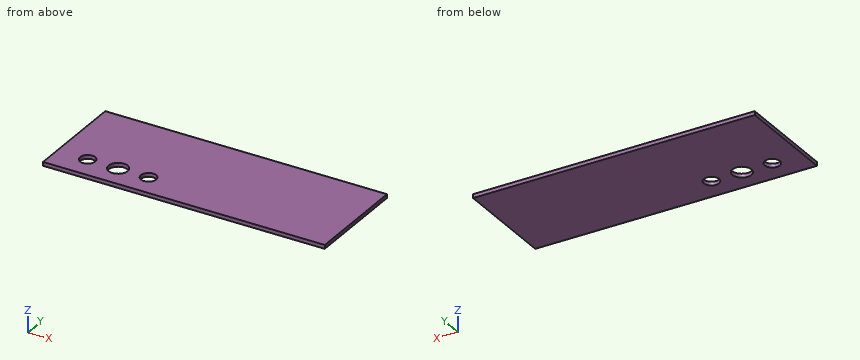
```python
from build123d import *

# Parameters (mm, degrees)
SKETCH1_W          = 234.95
SKETCH1_H          = 86.36
BASE_FLANGE1_DEPTH = 3.175
SKETCH11_R         = 7.9375
CUT_EXTRUDE3_DEPTH = 126.199715056
SKETCH13_R         = 6.35
CUT_EXTRUDE5_DEPTH = 126.199715056
SKETCH14_R         = 6.35
CUT_EXTRUDE6_DEPTH = 126.199715056


# Sheet-metal steps are written as plain solids
with BuildPart() as part:
    # Sketch1 → Base-Flange1 (new body)
    with BuildSketch(Plane.XY):
        Rectangle(SKETCH1_W, SKETCH1_H)
    extrude(amount=-BASE_FLANGE1_DEPTH)

    # Sketch11 → Cut-Extrude3 (cut, through all)
    with BuildSketch(Plane.XY):
        with Locations((-66.675, -23.495)):
            Circle(SKETCH11_R)
    extrude(amount=-CUT_EXTRUDE3_DEPTH, mode=Mode.SUBTRACT)

    # Sketch13 → Cut-Extrude5 (cut, through all)
    with BuildSketch(Plane.XY):
        with Locations((-41.275, -23.495)):
            Circle(SKETCH13_R)
    extrude(amount=-CUT_EXTRUDE5_DEPTH, mode=Mode.SUBTRACT)

    # Sketch14 → Cut-Extrude6 (cut, through all)
    with BuildSketch(Plane.XY):
        with Locations((-92.075, -23.495)):
            Circle(SKETCH14_R)
    extrude(amount=-CUT_EXTRUDE6_DEPTH, mode=Mode.SUBTRACT)


solid = part.part
```
Geometry: final body of the model. Coordinates: model frame, mm. Round coordinates to 2 decimals unless told otherwise and drop trailing zeros. Order: outer loops, then holes, each group sorted by start corner. A loop starts at its lowest first (then second) coordinate and runs counter-clockwise, first axis right, second up. Notation, with made-up numbers: (84, -27.5) -> (99, -27.5) arc R23 ccw to (99, 8.5) -> close; hole circle Ø9 at (78, -20.5). An arc over 180 degrees is marked (long way). Use one line per item in the form item = value. Start each with the question number.
1. Cut plane C-C (x = -95). Return the cut outline in (y, z) (3 decimals), then the cut area to 3 significant figures.
2. Cut plane B-B (z = -1.65). Count the separate pieces of the cut face and the enclosed holes in it, then the cut area to 3 significant figures.
3. Line query: probe 1 along X at (y, z) = (-23.5, -0.9) (1 decimal); probe 2 along X at (y, z) = (-20, -1.3) (3 decimals); probe 3 along Y at (x, z) = (-40.5, -2.6). Output: solid intervals per line, ascending.
4. Pin query (flat end, axial travel): pin 1 Ø7.5 at (x, y) = (-92.075, -23.495) entering from -Z. Return the tip coordinate at first contact, or that it passes through.
5. Cut plane A-A (x = -63.5). Return the cut outline in (y, z) (3 decimals).
Solution:
q1.outline = (-43.18, -3.175) -> (-29.131, -3.175) -> (-29.131, 0) -> (-43.18, 0) -> close; (-17.859, -3.175) -> (43.18, -3.175) -> (43.18, 0) -> (-17.859, 0) -> close
q1.area = 238 mm^2
q2.separate_pieces = 1
q2.enclosed_holes = 3
q2.area = 19,800 mm^2
q3.probe_1 = -117.5 to -98.4, -85.7 to -74.6, -58.7 to -47.6, -34.9 to 117.5
q3.probe_2 = -117.475 to -97.377, -86.773 to -73.802, -59.548 to -46.577, -35.973 to 117.475
q3.probe_3 = -43.18 to -29.8, -17.19 to 43.18
q4.pin_1 = through
q5.outline = (-43.18, -3.175) -> (-30.77, -3.175) -> (-30.77, 0) -> (-43.18, 0) -> close; (-16.22, -3.175) -> (43.18, -3.175) -> (43.18, 0) -> (-16.22, 0) -> close
